Could you check a few things on this model? Use its own coordinates, in mm. Face numbers are marked on the shaded views. A direction names the side the tool comes from. Give positions to 0.01 mm unless a question says otherwise; leave off trailing zeros. Order: outer loops, then holes, each group sorted by start corner. A loop starts at its lowest first (then second) coordinate and runs counter-clockwise, first axis right, second up. Notation, with made-up numbers: (66.25, -2.5) - (114.25, -2.5) arc R7 ccw to (114.25, 3.5) - close; hole circle Ø11 at (88, -34). An arc over 180 degrees is marked (long way). One line per question, with ' | ' between items. Start each with the question number.
1. Imagine slicing it at B-B (x = 16.5). Please give me the cut outline in (y, z) (3 decimals).
2. I need wall thicknesses on probe 1 along Y at (x, z) = (0, 8) (3 decimals); probe 2 along Y at (x, z) = (30.5, 11) (3 decimals); probe 3 along Y at (x, z) = (5, 6.75) (3 decimals). Which ranges of each line are inside material? Lowest first, please. Write a range as from..to.
3. Which directions (+Z, -Z, +X, -X, +Y, -Y) give clear straight access to the entire face, cutting with the end or side of a thin tool? Please do the marked faces 1, 2 and 3.
4. Imagine slicing it at A-A (z = 15.75). Please give me the cut outline in (x, y) (3 decimals).
5. For P1, Ø3, axis at x = -8, y = 53.5, coming from the -Z side; P2, Ø2.5, axis at y = 49.5, z = 4.5, coming from the -X side; P3, Ø1, axis at x = 14.5, z = 11.5, coming from the +Y side (3 decimals), each with a flat end and sliding along its axis, tell me the tip position at first contact or that it passes through.
6. If we mould it in two halves opening along Z, with no side actions, what happens to the marked faces 4, 5 and 6? For each: released by +Z, released by -Z, zero draft, split by the parting line, or undercut.
```python
from build123d import *

# Parameters (mm, degrees)
SKETCH1_W               = 65.35
SKETCH1_H               = 95.75
BOSS_EXTRUDE1_DEPTH     = 18.75
SKETCH2_R               = 1.36
CUT_EXTRUDE1_DEPTH      = 61.919896175
CUT_EXTRUDE_THIN1_START = -1
CUT_EXTRUDE_THIN1_DEPTH = 1
SKETCH5_W               = 19
SKETCH5_H               = 3
BOSS_EXTRUDE2_DEPTH     = 18.75
BOSS_EXTRUDE3_DEPTH     = 1.85


# Read off the part's stored shape, not the designer's step: Cut-Extrude-Thin1
with BuildPart() as part:
    # Sketch1 → Boss-Extrude1 (new body)
    with BuildSketch(Plane.XY):
        Rectangle(SKETCH1_W, SKETCH1_H)
    extrude(amount=BOSS_EXTRUDE1_DEPTH)

    # Sketch2 → Cut-Extrude1 (cut, through all)
    with BuildSketch(Plane.XY.offset(18.75)):
        with Locations((0, 39.675)):
            Circle(SKETCH2_R)
        with Locations((0, -5.125)):
            Circle(SKETCH2_R)
    extrude(amount=-CUT_EXTRUDE1_DEPTH, mode=Mode.SUBTRACT)

    # Cut-Extrude-Thin1 outline → Cut-Extrude-Thin1 (cut)
    with BuildSketch(Plane.XY.offset(18.75).offset(CUT_EXTRUDE_THIN1_START)):
        Polygon((1, 0), (1, 24.947040452), (9.414099592, 24.947040452), (0, 34.361140044), (-9.414099592, 24.947040452), (-1, 24.947040452), (-1, 0), align=None)
        Polygon((-4.585672467, 26.947040452), (-1, 30.532712919), (-1, 26.947040452), align=None, mode=Mode.SUBTRACT)
        Polygon((1, 26.947040452), (1, 30.532712919), (4.585672467, 26.947040452), align=None, mode=Mode.SUBTRACT)
    extrude(amount=CUT_EXTRUDE_THIN1_DEPTH, mode=Mode.SUBTRACT)

    # Sketch5 → Boss-Extrude2 (add)
    with BuildSketch(Plane.XY.offset(18.75)):
        with Locations((0, 49.375)):
            Rectangle(SKETCH5_W, SKETCH5_H)
    extrude(amount=-BOSS_EXTRUDE2_DEPTH)

    # Sketch6 → Boss-Extrude3 (add)
    with BuildSketch(Plane.XY.offset(18.75)):
        Polygon((-32.675, 57.875), (32.675, 57.875), (32.675, 47.875), (9.5, 47.875), (9.5, 50.875), (-9.5, 50.875), (-9.5, 47.875), (-32.675, 47.875), align=None)
    extrude(amount=-BOSS_EXTRUDE3_DEPTH)


solid = part.part
```
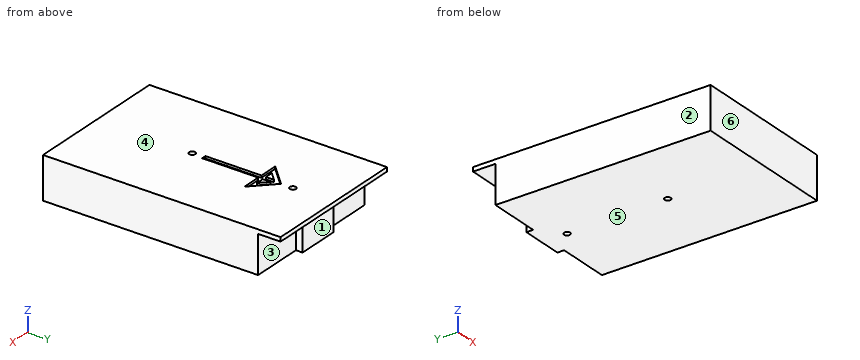
Results found:
1) outline: (-47.875, 0) - (47.875, 0) - (47.875, 16.9) - (57.875, 16.9) - (57.875, 18.75) - (-47.875, 18.75) - close
2) probe 1: y = -47.875..-6.485, -3.765..38.315, 41.035..50.875 | probe 2: y = -47.875..47.875 | probe 3: y = -47.875..50.875
3) face 1: -Z, +X, -X, +Y | face 2: +Z, -Z, -X, +Y, -Y | face 3: -Z, +X, +Y
4) outline: (-32.675, -47.875) - (32.675, -47.875) - (32.675, 47.875) - (9.5, 47.875) - (9.5, 50.875) - (-9.5, 50.875) - (-9.5, 47.875) - (-32.675, 47.875) - close; hole circle Ø2.72 at (0, -5.125); hole circle Ø2.72 at (0, 39.675)
5) P1: stops at z = 16.9 | P2: stops at x = -9.5 | P3: stops at y = 47.875
6) face 4: released by +Z | face 5: released by -Z | face 6: zero draft
